Could you check a few things on this model? Use its own coordinates, in mm. A direction names the side the tool comes from. Coordinates: 2 decimals unless noted, no trailing zeros. Loops run counter-clockwise (first coordinate to the right, second up) from the corner with the lowest first, then second, coordinate; pieces in that order, holes last. Notation, with made-up numbers: M 71,45.25 L 79,45.25 A12 ccw 79,61.25 Z; hole C 60.5,63 d4. An arc over 180 degrees is marked long. Return JSON: item names as keys, results as strings. Group by question number.
from build123d import *

# Parameters (mm, degrees)
F0_W     = 110
F0_H     = 60
F1_DEPTH = 50
F2_W     = 100
F2_H     = 50
F3_DEPTH = 25
F5_W     = 10
F5_H     = 15
F5_H_2   = 14.999788
F5_H_3   = 14.999776
F5_H_4   = 14.999488
F5_H_5   = 14.999479
F5_H_6   = 14.999535
F6_DEPTH = 15


with BuildPart() as f1:
    # F0 (on Top) → F1 (new body)
    with BuildSketch(Plane.XY):
        with Locations((1.447366, 11.055018)):
            Rectangle(F0_W, F0_H)
    extrude(amount=F1_DEPTH)

    # F2 (on face) → F3 (cut)
    with BuildSketch(Plane(origin=(0, 0, 0), x_dir=(1, 0, 0), z_dir=(0, 0, -1))):
        with Locations((1.447366, -11.055018)):
            Rectangle(F2_W, F2_H)
    extrude(amount=-F3_DEPTH, mode=Mode.SUBTRACT)

    # F5 (on face) → F6 (cut)
    with BuildSketch(Plane.XY.offset(50)):
        with Locations((-43.552634, 23.555018)):
            Rectangle(F5_W, F5_H)
        with Locations((-28.552634, 23.555124)):
            Rectangle(F5_W, F5_H_2)
        with Locations((-13.552634, 23.555018)):
            Rectangle(F5_W, F5_H)
        with Locations((1.447366, 23.55513)):
            Rectangle(F5_W, F5_H_3)
        with Locations((16.447366, 23.555274)):
            Rectangle(F5_W, F5_H_4)
        with Locations((31.447366, 23.555279)):
            Rectangle(F5_W, F5_H_5)
        with Locations((46.447366, 23.55525)):
            Rectangle(F5_W, F5_H_6)
        with Locations((-43.552634, -1.444982)):
            Rectangle(F5_W, F5_H)
        with Locations((-28.552634, -1.444982)):
            Rectangle(F5_W, F5_H)
        with Locations((-13.552634, -1.444982)):
            Rectangle(F5_W, F5_H)
        with Locations((1.447366, -1.444982)):
            Rectangle(F5_W, F5_H)
        with Locations((16.447366, -1.444982)):
            Rectangle(F5_W, F5_H)
        with Locations((31.447366, -1.444982)):
            Rectangle(F5_W, F5_H)
        with Locations((46.447366, -1.444982)):
            Rectangle(F5_W, F5_H)
    extrude(amount=-F6_DEPTH, mode=Mode.SUBTRACT)


solid = f1.part
(1) Imagine slicing it at A-A, the plane x = -32. Write out the boundary of the cut face in (y, z).
(2) We'd pull the mould along X, two halves only. Please class faces 3 (the face through (31, -8.945, 43)), 4 (the face through (-44, 31.055, 43)), 5 (the face through (1, 41.055, 25)): +X half, -X half, draft (parallel to the pull), parting line (faces both ways), or undercut.
(3) Imagine slicing it at B-B, the plane z = 23.5. Write out the boundary of the cut face in (x, y), then the cut area to 3 significant figures.
(4) For faces 1 (the face through (1, 36.055, 12)), 2 (the face through (-48.553, 23, 43)), which set-ups out of +Z, -Z, +X, -X, +Y, -Y let a thin tool reach every point of the face, with its end or its side?
(5) If I drill on L1, parallel to Y at x = 36, z = 40.5; L2, parallel to X at y = 27, z = 15; L3, parallel to Y at x = 19, z = 9, over which ranges is the centre line in solid material (lowest first)? Write a range as [from, to].
(6) Imagine slicing it at C-C, the plane z = 42. Count the separate pieces of the cut face and the enclosed holes in it, then the cut area to 3 significant figures.
(7) Will this pin go through, and if not, where does the flat tip stop? P1, Ø1, axis at x = -25.5, y = 9, coming from the -Z side.
Checks:
{
 "1": {"outline": "M -18.94,0 L -13.94,0 L -13.94,25 L 36.06,25 L 36.06,0 L 41.06,0 L 41.06,50 L 31.06,50 L 31.06,35 L 16.06,35 L 16.06,50 L 6.06,50 L 6.06,35 L -8.94,35 L -8.94,50 L -18.94,50 Z"},
 "2": {"face 3": "undercut", "face 4": "undercut", "face 5": "draft"},
 "3": {"outline": "M -53.55,-18.94 L 56.45,-18.94 L 56.45,41.06 L -53.55,41.06 Z; hole M -48.55,-13.94 L 51.45,-13.94 L 51.45,36.06 L -48.55,36.06 Z", "area": "1,600 mm²"},
 "4": {"face 1": "-Z", "face 2": "+Z"},
 "5": {"L1": "[-18.94, -8.94], [6.06, 16.06], [31.06, 41.06]", "L2": "[-53.55, -48.55], [51.45, 56.45]", "L3": "[-18.94, -13.94], [36.06, 41.06]"},
 "6": {"separate pieces": "1", "enclosed holes": "14", "area": "4,500 mm²"},
 "7": {"P1": "z = 25"}
}
